Verification items for the finished model (mm, model axes). Give positions to 0.01 mm unless a question says otherwise; leave off trailing zeros. Order: outer loops, then holes, each group sorted by start corner. A loop starts at its lowest first (then second) coordinate and runs counter-clockwise, first axis right, second up. Notation, with made-up numbers: M 12.25,47 L 41.25,47 A14 cw 41.25,54 Z; hole C 60,-8.75 d11. An arc over 180 degrees is marked long. Answer as a JSON object with one key per item and string values.
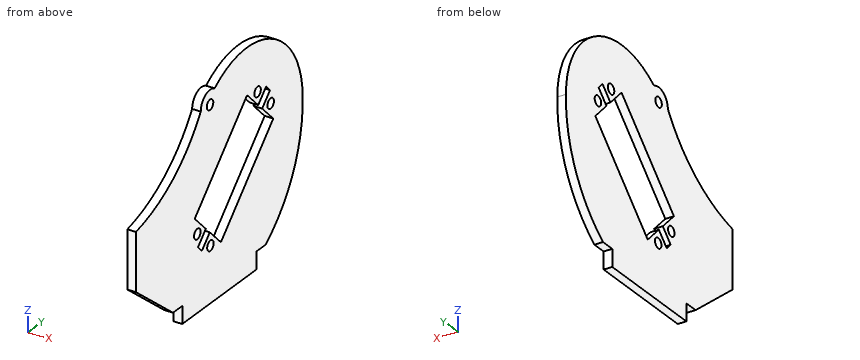
```python
from build123d import *

# Parameters (mm, degrees)
CROQUIS1_R              = 1.75
SALIENTE_EXTRUIR1_DEPTH = 3


with BuildPart() as part:
    # Croquis1 → Saliente-Extruir1 (new body)
    with BuildSketch(Plane(origin=(0, 0, 0), x_dir=(0, 0, -1), z_dir=(1, 0, 0))):
        with BuildLine():
            Line((4.142135624, -60), (24.142135624, -60))
            Line((24.142135624, -60), (40, -40))
            Line((40, -40), (40, -35))
            Line((40, -35), (46, -35))
            Line((46, -35), (46, 5))
            Line((46, 5), (40, 5))
            Line((40, 5), (40, 10))
            ThreePointArc((40, 10), (22.503199777, 25.006399554), (0, 30))
            ThreePointArc((0, 30), (-26.700709952, 13.677429877), (-24.346472536, -17.528527464))
            ThreePointArc((-24.346472536, -17.528527464), (-24.321884003, -22.514223272), (-20, -25))
            ThreePointArc((-20, -25), (-4.291896326, -39.991262484), (4.142135624, -60))
        make_face()
        with Locations((-12.730077402, 5.654698909)):
            Circle(CROQUIS1_R, mode=Mode.SUBTRACT)
        with Locations((-5.658477353, 12.726298958)):
            Circle(CROQUIS1_R, mode=Mode.SUBTRACT)
        with Locations((26.870057685, -19.798989873)):
            Circle(CROQUIS1_R, mode=Mode.SUBTRACT)
        with Locations((19.797157185, -26.871890373)):
            Circle(CROQUIS1_R, mode=Mode.SUBTRACT)
        with Locations((-20, -20)):
            Circle(CROQUIS1_R, mode=Mode.SUBTRACT)
        Polygon((-14.142135624, 0), (14.142135624, -28.284271247), (20.150710576, -22.275696296), (24.393351263, -26.518336983), (26.516504294, -24.395183951), (22.273863607, -20.152543264), (28.284271247, -14.142135624), (0, 14.142135624), (-6.01040764, 8.131727984), (-10.253048327, 12.374368671), (-12.374368671, 10.253048327), (-8.131727984, 6.01040764), align=None, mode=Mode.SUBTRACT)
    extrude(amount=SALIENTE_EXTRUIR1_DEPTH)


solid = part.part
```
Q1. Section check B-B on x = 0.8. Record the cut outline in (y, z), then the cut area to 3 significant figures.
Resolved:
{"outline": "M -60,-24.14 L -40,-40 L -35,-40 L -35,-46 L 5,-46 L 5,-40 L 10,-40 A47.46 ccw 30,0 A30 ccw -17.53,24.35 A5 ccw -25,20 A53.36 cw -60,-4.14 Z; hole C -26.87,-19.8 d3.5; hole M -28.28,-14.14 L -22.28,-20.15 L -26.52,-24.39 L -24.4,-26.52 L -20.15,-22.27 L -14.14,-28.28 L 14.14,0 L 8.13,6.01 L 12.37,10.25 L 10.25,12.37 L 6.01,8.13 L 0,14.14 Z; hole C -20,20 d3.5; hole C -19.8,-26.87 d3.5; hole C 5.65,12.73 d3.5; hole C 12.73,5.66 d3.5", "area": "4,100 mm²"}
Q2. Section check A-A on y = -16.5. Record the cut outline in (x, z).
Resolved:
{"outline": "M 0,-46 L 3,-46 L 3,-25.93 L 0,-25.93 Z; M 0,-2.36 L 3,-2.36 L 3,25.05 L 0,25.05 Z"}
Q3. Section check C-C on z = -2. Record the cut outline in (x, y), then the cut area to 3 significant figures.
Resolved:
{"outline": "M 0,-52.24 L 3,-52.24 L 3,-16.14 L 0,-16.14 Z; M 0,12.14 L 3,12.14 L 3,30.01 L 0,30.01 Z", "area": "162 mm²"}
Q4. Section check D-D on y = 17.5. Record the cut outline in (x, z).
Resolved:
{"outline": "M 0,-33.39 L 3,-33.39 L 3,24.37 L 0,24.37 Z"}
Q5. Material ranges on L1, parallel to Y at x = 0.4, z = -19.5; L2, parallel to Z at x = 2.2, y = 12.5; L3, parallel to Y at x = 1.4, z = -22.5, recorded low to high.
Resolved:
{"L1": "y = -60 to -28.6, -25.15 to -22.93, -5.36 to 26.38", "L2": "z = -38.1 to -1.64, 1.64 to 3.92, 7.39 to 27.27", "L3": "y = -60 to -24.62, -20.38 to -19.93, -8.36 to 25.01"}
Q6. Gauge pin test, flat ends, axial feed: pin 1 Ø1.5 at (x, z) = (1, -42) entering from -Y; pin 2 Ø6 at (y, z) = (5.5, -1) entering from -X; pin 3 Ø1 at (x, y) = (2, -12) entering from +Z. Record the tip position at first contact, or that the pin passes through.
Resolved:
{"pin 1": "stops at y = -35", "pin 2": "passes through", "pin 3": "stops at z = 27.71"}
